```python
from build123d import *

# Parameters (mm, degrees)
SKETCH1_W                        = 76.2
SKETCH1_H                        = 31.75
EXTRUDE1_DEPTH                   = 3.175
F_27_64_0_42188_DIAMETER_HOLE1_D = 10.715752


with BuildPart() as part:
    # Sketch1 → Extrude1 (new, symmetric)
    with BuildSketch(Plane.XY):
        Rectangle(SKETCH1_W, SKETCH1_H)
    extrude(amount=EXTRUDE1_DEPTH, both=True)

    # 27/64 (0.42188) Diameter Hole1 (through all)
    with Locations(Plane(origin=(25.4, 0, 3.175), x_dir=(1, 0, 0), z_dir=(0, 0, 1))):
        with Locations((0, 0)):
            Hole(F_27_64_0_42188_DIAMETER_HOLE1_D / 2)


solid = part.part
```
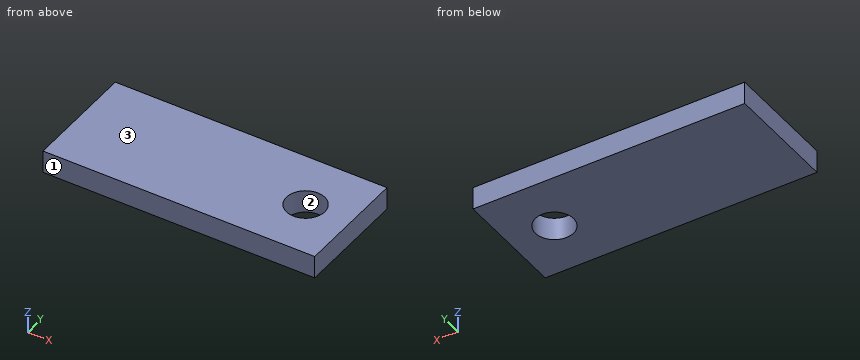
The model under review builds one solid part; all positions refer to its coordinate system, in mm. Face numbers are marked on the shaded views. Give positions to 0.01 mm unless a question says otherwise; leave off trailing zeros. Write each loop counter-clockwise with the first axis right and the second up, starting at its lowest first coordinate (ties: lowest second). Pieces come first, ordered by that corner, then holes. Notation, with made-up numbers: M -9.75,60.5 L 35.25,60.5 A14 cw 35.25,73.5 Z; hole C -19,4 d3. An arc over 180 degrees is marked long. Write item = value, one per line. Start each with the question number.
Q1. Mouldability with a two-part tool opening along Y and no side actions: class the marked faces 1, 2 and 3 as released by +Y, released by -Y, zero draft, split by the parting line, or undercut.
Q2. We need section A-A (y = 0). State the section outline as (x, z) points (3 decimals).
Q3. We need section B-B (x = 25.4). State the section outline as (y, z) points (3 decimals).
Q4. We need section C-C (z = 1.25). State the section outline as (x, y) points (3 decimals).
Q5. For line 1 (Y direction, x = 25.4, z = 0.5) (3 decimals); line 2 (X direction, y = -1, z = -2.5); line 3 (Y direction, x = 20.5, z = 1.25) (3 decimals), list the stretches that pass through material, from the lowest coordinate up.
Result set:
q1.face_1 = released by -Y
q1.face_2 = undercut
q1.face_3 = zero draft
q2.outline = M -38.1,-3.175 L 20.042,-3.175 L 20.042,3.175 L -38.1,3.175 Z; M 30.758,-3.175 L 38.1,-3.175 L 38.1,3.175 L 30.758,3.175 Z
q3.outline = M -15.875,-3.175 L -5.358,-3.175 L -5.358,3.175 L -15.875,3.175 Z; M 5.358,-3.175 L 15.875,-3.175 L 15.875,3.175 L 5.358,3.175 Z
q4.outline = M -38.1,-15.875 L 38.1,-15.875 L 38.1,15.875 L -38.1,15.875 Z; hole C 25.4,0 d10.716
q5.line_1 = -15.875 to -5.358, 5.358 to 15.875
q5.line_2 = -38.1 to 20.14, 30.66 to 38.1
q5.line_3 = -15.875 to -2.167, 2.167 to 15.875
